Source: three-view drawing plus pictorial views. Frame: mm from the lowest corner of the part. A direction names the side the tool comes from. Round coordinates to 2 decimals unless told otherwise and drop trailing zeros. Loops run counter-clockwise (first coordinate to the right, second up) from the corner with the lowest first, then second, coordinate; pieces in that order, holes last. Notation, with made-up numbers: (-27.5, 19.5) -> (-0.5, 19.5) arc R19 ccw to (-0.5, 38.5) -> close; hole circle Ø6 at (-38, -7). An arc over 180 degrees is marked (long way). One line per question, with ' | ' between items. Start each with the question number.
Q1. Cut plane B-B on z = 22. Return loops of the section in (x, y).
Q2. Cut plane A-A on x = 478. Return loops of the section in (y, z), and give its area (3 significant figures).
Q3. Material intervals for L1, parallel to Y at x = 272, z = 24.5, sorted ascending.
Q4. Contact query for flat-ended pins moving along their axis: P1, Ø8.5, axis at x = 129.159, y = 25.4, coming from the +Z side; P2, Ø10, axis at x = 15.875, y = 25.4, coming from the -Z side; P3, Ø4, axis at x = 332, z = 37.5, coming from the -Y side. Output: stop coordinate, or through.
Q5. Access query for the marked faces 1 and 2. Directions: +Z, -Z, +X, -X, +Y, -Y. A direction counts if a zero-diameter tool reaches every point of the face in a straight line with its end or side. Return the directions, or none.
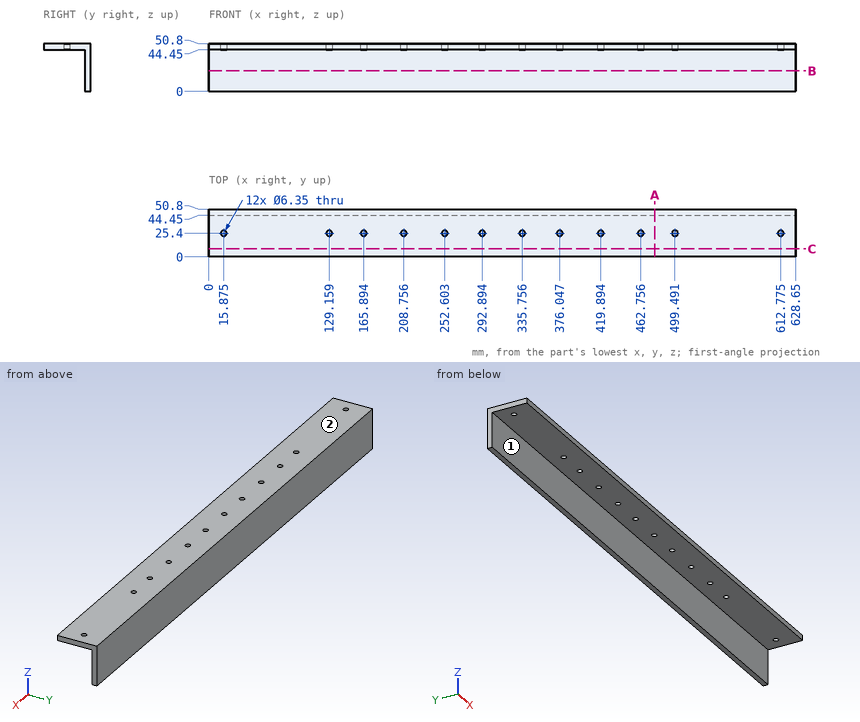
Results:
1) outline: (0, 44.45) -> (628.65, 44.45) -> (628.65, 50.8) -> (0, 50.8) -> close
2) outline: (0, 44.45) -> (44.45, 44.45) -> (44.45, 0) -> (50.8, 0) -> (50.8, 50.8) -> (0, 50.8) -> close | area: 605 mm^2
3) L1: 44.45 to 50.8
4) P1: z = 50.8 | P2: z = 44.45 | P3: y = 44.45
5) face 1: -Z, +X, -X, -Y | face 2: +Z, +X, -X, +Y, -Y
